Could you check a few things on this model? Use its own coordinates, in mm. A direction names the side the tool comes from. Coordinates: 2 decimals unless noted, no trailing zeros. Loops run counter-clockwise (first coordinate to the right, second up) from the corner with the lowest first, then second, coordinate; pieces in that order, holes last. Notation, with made-up numbers: (82.25, 30.25) - (88.25, 30.25) arc R15 ccw to (88.25, 42.25) - close; hole circle Ø4 at (84.5, 11.5). An arc over 180 degrees is marked (long way). One line per item, written item: value. Start each with the question number.
(1) On a 3-axis mill with a long thin cutter (end or side, diameter ignored), from which of +Z, -Z, +X, -X, +Y, -Y can I reach the whole of each face in a straight line? I mean faces 1 (the face through (80, 12, 29)), 2 (the face through (38, 2, 52)), 3 (the face through (8, 14, 8)). Say none if no direction works.
(2) If we section it at A-A on x = 31: Write out the boundary of the cut face in (y, z).
(3) If we section it at D-D on z = 51: Write out the boundary of the cut face in (x, y).
(4) If I drill on line 1 along Z through (x, y) = (51.5, 8.5); line 2 along Z through (x, y) = (16.5, 11); line 3 along Y through (x, z) = (39, 49), over which ranges is the centre line in solid material (lowest first)? Write a range as from..to.
(5) If we section it at B-B on y = 19: Count the separate pieces of the cut face and the enclosed holes in it, then the cut area to 3 significant figures.
(6) If we mould it in two halves opening along X, with no side actions, what happens to faces 4 (the face through (67.18, 13.79, 25.77)), 5 (the face through (18, 18, 49)), 6 (the face through (16, 18, 11)), 7 (the face through (70.73, 3.31, 28.59))? For each: pulls with the +X half, pulls with the -X half, needs draft (parallel to the pull), parting line crosses it, or undercut.
(7) If we section it at C-C on z = 25.5: Write out the boundary of the cut face in (x, y), then the cut area to 3 significant figures.
(8) I'm going to push flat-ended pins straight in: P1, Ø13, axis at x = 11, y = 10, coming from the +Z side; P2, Ø2, axis at y = 27.5, z = 33.5, coming from the -X side; P3, Ø1.8, axis at y = 9.5, z = 48, coming from the -X side. Where does each tip first touch, or does it pass through?
```python
from build123d import *

# Parameters (mm, degrees)
SKETCH1_R           = 7.5
BOSS_EXTRUDE1_DEPTH = 58
CUT_EXTRUDE1_DEPTH  = 107.60206377
SKETCH3_R           = 7
CUT_EXTRUDE2_DEPTH  = 107.60206377
SKETCH5_W           = 17.33939444
SKETCH5_H           = 15
CUT_EXTRUDE3_DEPTH  = 107.602063899
CUT_EXTRUDE4_START  = -12
SKETCH6_R           = 7.5
CUT_EXTRUDE4_DEPTH  = 12
CUT_EXTRUDE5_START  = -6
CUT_EXTRUDE5_DEPTH  = 6


with BuildPart() as part:
    # Sketch1 → Boss-Extrude1 (new body)
    with BuildSketch(Plane.XY):
        with BuildLine():
            Line((0, 0), (65, 0))
            Line((65, 0), (80, 8.660254038))
            Line((80, 8.660254038), (80, 31.339745962))
            Line((80, 31.339745962), (65, 40))
            Line((65, 40), (36.66060556, 40))
            ThreePointArc((36.66060556, 40), (16.66060556, 35.82575695), (0, 24))
            Line((0, 24), (0, 0))
        make_face()
        with Locations(Location((34, 19, 0), (0, 0, 180))):
            Circle(SKETCH1_R, mode=Mode.SUBTRACT)
    extrude(amount=BOSS_EXTRUDE1_DEPTH)

    # Sketch2 → Cut-Extrude1 (cut, through all)
    with BuildSketch(Plane.XZ):
        Polygon((80, 58), (65, 58), (80, 43), align=None)
        Polygon((80, 15), (65, 0), (80, 0), align=None)
    extrude(amount=-CUT_EXTRUDE1_DEPTH, mode=Mode.SUBTRACT)

    # Sketch3 → Cut-Extrude2 (cut, through all)
    with BuildSketch(Plane(origin=(80, 0, 0), x_dir=(0, 0, -1), z_dir=(1, 0, 0))):
        with Locations((-29, 20)):
            Circle(SKETCH3_R)
    extrude(amount=-CUT_EXTRUDE2_DEPTH, mode=Mode.SUBTRACT)

    # Sketch5 → Cut-Extrude3 (cut, through all)
    with BuildSketch(Plane(origin=(0, 40, 0), x_dir=(1, 0, 0), z_dir=(0, 1, 0))):
        Polygon((16, -8), (0, -8), (0, -29), (36.66060556, -29), (36.66060556, -14), (16, -14), align=None)
        with Locations((45.33030278, -21.5)):
            Rectangle(SKETCH5_W, SKETCH5_H)
        with Locations((45.33030278, -36.5)):
            Rectangle(SKETCH5_W, SKETCH5_H)
        Polygon((36.66060556, -29), (0, -29), (0, -50), (16, -50), (16, -44), (36.66060556, -44), align=None)
    extrude(amount=-CUT_EXTRUDE3_DEPTH, mode=Mode.SUBTRACT)

    # Sketch6 → Cut-Extrude4 (cut)
    with BuildSketch(Plane.XY.offset(58).offset(CUT_EXTRUDE4_START)):
        with BuildLine():
            Line((18, 34.224221872), (18, 2))
            Line((18, 2), (63, 2))
            Line((63, 2), (63, 38))
            Line((63, 38), (36.66060556, 38))
            ThreePointArc((36.66060556, 38), (27.141221384, 37.046586751), (18, 34.224221872))
        make_face()
        with Locations(Location((34, 19, 0), (0, 0, 180))):
            Circle(SKETCH6_R, mode=Mode.SUBTRACT)
    extrude(amount=CUT_EXTRUDE4_DEPTH, mode=Mode.SUBTRACT)

    # Sketch7 → Cut-Extrude5 (cut)
    with BuildSketch(Plane.XY.offset(58).offset(CUT_EXTRUDE5_START)):
        with BuildLine():
            Line((18, 2), (18, 34.224221872))
            ThreePointArc((18, 34.224221872), (9.117311148, 29.311155325), (1.466424222, 22.64))
            Line((1.466424222, 22.64), (0, 21.058823529))
            Line((0, 21.058823529), (0, 2))
            Line((0, 2), (18, 2))
        make_face()
    extrude(amount=CUT_EXTRUDE5_DEPTH, mode=Mode.SUBTRACT)


solid = part.part
```
Values:
1. face 1: +Z, -Z, +X, +Y, -Y
1. face 2: +Z
1. face 3: -X, +Y, -Y
2. outline: (0, 0) - (12.13, 0) - (12.13, 14) - (0, 14) - close; (0, 44) - (12.13, 44) - (12.13, 46) - (2, 46) - (2, 58) - (0, 58) - close; (25.87, 0) - (39.68, 0) - (39.68, 14) - (25.87, 14) - close; (25.87, 44) - (39.68, 44) - (39.68, 58) - (37.67, 58) - (37.67, 46) - (25.87, 46) - close
3. outline: (0, 0) - (65, 0) - (72, 4.04) - (72, 35.96) - (65, 40) - (36.66, 40) arc R50 ccw to (0, 24) - close; hole (18, 2) - (63, 2) - (63, 38) - (36.66, 38) arc R48 ccw to (18, 34.22) - close
4. line 1: z = 0..14, 44..46
4. line 2: z = 0..14, 44..52
4. line 3: y = 0..2, 38..40
5. separate pieces: 4
5. enclosed holes: 0
5. area: 1,350 mm2
6. face 4: needs draft
6. face 5: undercut
6. face 6: pulls with the -X half
6. face 7: pulls with the +X half
7. outline: (54, 0) - (65, 0) - (80, 8.66) - (80, 13.94) - (54, 13.94) - close; (54, 26.06) - (80, 26.06) - (80, 31.34) - (65, 40) - (54, 40) - close
7. area: 595 mm2
8. P1: stops at z = 52
8. P2: stops at x = 54
8. P3: stops at x = 16
